from build123d import *

# Parameters (mm, degrees)
SKETCH1_W             = 152.4
SKETCH1_H             = 152.4
SKETCH1_W_2           = 146.05
SKETCH1_H_2           = 146.05
BOSS_EXTRUDE1_DEPTH   = 127
SKETCH2_W             = 146.05
SKETCH2_H             = 146.05
BOSS_EXTRUDE2_DEPTH   = 3.175
SKETCH3_W             = 146.05
SKETCH3_H             = 146.05
BOSS_EXTRUDE3_DEPTH   = 3.175
SKETCH4_W             = 50.8
SKETCH4_H             = 25.4
BOSS_EXTRUDE4_DEPTH   = 25.4
BOSS_EXTRUDE4_2_DEPTH = 25.4
SKETCH7_R             = 6.35
BOSS_EXTRUDE5_DEPTH   = 25.4
SKETCH8_R             = 6.35
BOSS_EXTRUDE6_DEPTH   = 19.05
SKETCH9_R             = 6.35
BOSS_EXTRUDE7_DEPTH   = 19.05


with BuildPart() as part:
    # Sketch1 → Boss-Extrude1 (new, symmetric)
    with BuildSketch(Plane.XY):
        Rectangle(SKETCH1_W, SKETCH1_H)
        Rectangle(SKETCH1_W_2, SKETCH1_H_2, mode=Mode.SUBTRACT)
    extrude(amount=BOSS_EXTRUDE1_DEPTH, both=True)

    # Sketch2 → Boss-Extrude2 (add)
    with BuildSketch(Plane.XY.offset(127)):
        Rectangle(SKETCH2_W, SKETCH2_H)
    extrude(amount=-BOSS_EXTRUDE2_DEPTH)

    # Sketch3 → Boss-Extrude3 (add)
    with BuildSketch(Plane(origin=(0, 0, -127), x_dir=(-1, 0, 0), z_dir=(0, 0, -1))):
        Rectangle(SKETCH3_W, SKETCH3_H)
    extrude(amount=-BOSS_EXTRUDE3_DEPTH)

    # Sketch6 → Revolve2 (revolve)
    with BuildSketch(Plane(origin=(0, 0, -101.6), x_dir=(-1, 0, 0), z_dir=(0, 0, -1))):
        with BuildLine():
            Line((0, -76.2), (0, -127))
            ThreePointArc((0, -127), (17.960512242, -119.560512242), (25.4, -101.6))
            Line((25.4, -101.6), (9.525, -101.6))
            Line((9.525, -101.6), (9.525, -76.2))
            Line((9.525, -76.2), (0, -76.2))
        make_face()
    revolve(axis=Axis((0, -76.2, -101.6), (0, -1, 0)))

    # Sketch7 → Boss-Extrude5 (add)
    with BuildSketch(Plane(origin=(0, 76.2, 0), x_dir=(1, 0, 0), z_dir=(0, 1, 0))):
        with Locations(Location((0, 0, 0), (0, 0, 90))):
            Circle(SKETCH7_R)
    extrude(amount=BOSS_EXTRUDE5_DEPTH)


with BuildPart() as body_2:
    # Sketch4 → Boss-Extrude4 (new body)
    with BuildSketch(Plane.XZ.offset(76.2)):
        with Locations((50.8, 88.9)):
            Rectangle(SKETCH4_W, SKETCH4_H)
    extrude(amount=BOSS_EXTRUDE4_DEPTH)


    add(part.part)  # Boss-Extrude6 merges part
    # Sketch8 → Boss-Extrude6 (add)
    with BuildSketch(Plane(origin=(76.2, 0, 0), x_dir=(0, 0, -1), z_dir=(1, 0, 0))):
        with Locations(Location((-88.9, -88.9, 0), (0, 0, 180))):
            Circle(SKETCH8_R)
    extrude(amount=BOSS_EXTRUDE6_DEPTH)


with BuildPart() as body_3:
    # Sketch4 → Boss-Extrude4 2 (new body)
    with BuildSketch(Plane.XZ.offset(76.2)):
        with Locations((-50.8, 88.9)):
            Rectangle(SKETCH4_W, SKETCH4_H)
    extrude(amount=BOSS_EXTRUDE4_2_DEPTH)


    add(body_2.part)  # Boss-Extrude7 merges body 2
    # Sketch9 → Boss-Extrude7 (add)
    with BuildSketch(Plane.ZY.offset(76.2)):
        with Locations(Location((88.9, -88.9, 0), (0, 0, 180))):
            Circle(SKETCH9_R)
    extrude(amount=BOSS_EXTRUDE7_DEPTH)


solid = body_3.part
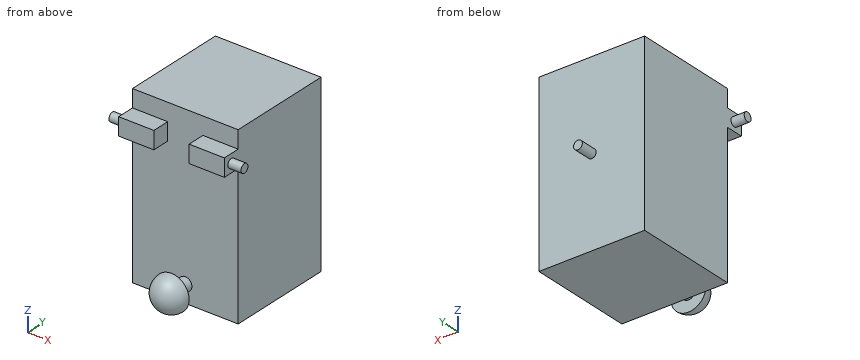
Verification items for the finished model (mm, model axes). Give positions to 0.01 mm unless a question says otherwise; leave off trailing zeros. Loops run counter-clockwise (first coordinate to the right, second up) from the corner with the lowest first, then second, coordinate; pieces in that order, holes last.
1. Cross-section at A-A on z = 50.5. Record the cut outline in (x, y) (3 decimals).
Derived:
outline: (-76.2, -76.2) - (76.2, -76.2) - (76.2, 76.2) - (-76.2, 76.2) - close; hole (-73.025, -73.025) - (73.025, -73.025) - (73.025, 73.025) - (-73.025, 73.025) - close
2. Cross-section at B-B on y = -11. Record the cut outline in (x, z) (3 decimals).
Derived:
outline: (-76.2, -127) - (76.2, -127) - (76.2, 127) - (-76.2, 127) - close; hole (-73.025, -123.825) - (73.025, -123.825) - (73.025, 123.825) - (-73.025, 123.825) - close
3. Cross-section at D-D on y = -88.9. Record the cut outline in (x, z) (3 decimals).
Derived:
outline: (-95.25, 82.55) - (-76.2, 82.55) - (-76.2, 76.2) - (-25.4, 76.2) - (-25.4, 101.6) - (-76.2, 101.6) - (-76.2, 95.25) - (-95.25, 95.25) - close; circle Ø19.05 at (0, -101.6); (25.4, 76.2) - (76.2, 76.2) - (76.2, 82.55) - (95.25, 82.55) - (95.25, 95.25) - (76.2, 95.25) - (76.2, 101.6) - (25.4, 101.6) - close
4. Go/stop test with flat-tipped pins: P1, Ø2, axis at y = -76.5, z = 64, coming from the -X side; P2, Ø1, axis at x = -34.5, z = -40.5, coming from the -Y side; P3, Ø10, axis at x = 40.5, z = 88, coming from the -Y side. Record where each tip stops, or that it passes through.
Derived:
P1: stops at x = -76.2
P2: stops at y = -76.2
P3: stops at y = -101.6
5. Cross-section at C-C on x = 0. Record the cut outline in (y, z) (3 decimals).
Derived:
outline: (-101.6, -127) - (-101.6, -111.125) - (-76.2, -111.125) - (-76.2, -127) - (76.2, -127) - (76.2, -6.35) - (101.6, -6.35) - (101.6, 6.35) - (76.2, 6.35) - (76.2, 127) - (-76.2, 127) - (-76.2, -92.075) - (-101.6, -92.075) - (-101.6, -76.2) arc R25.4 ccw to start; hole (-73.025, -123.825) - (73.025, -123.825) - (73.025, 123.825) - (-73.025, 123.825) - close
6. Material ranges on probe 1 along Y at (x, z) = (68, -11) (3 decimals); probe 2 along Z at (x, y) = (19, 10) (3 decimals), recorded low to high.
Derived:
probe 1: y = -76.2 to -73.025, 73.025 to 76.2
probe 2: z = -127 to -123.825, 123.825 to 127
